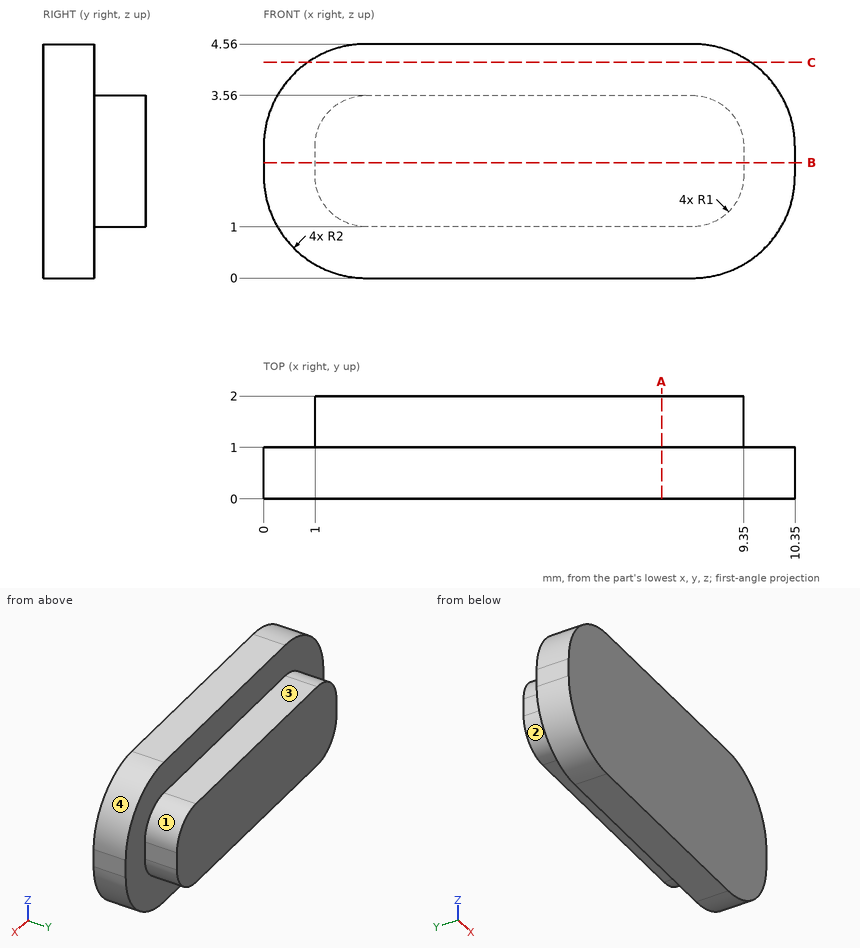
Print and shaded views of the part. All mm, measured from the part's lowest x, y and z. A direction names the side the tool comes from. Coordinates: 2 decimals unless noted, no trailing zeros. Order: outer loops, then holes, each group sorted by start corner. A loop starts at its lowest first (then second) coordinate and runs counter-clockwise, first axis right, second up. Notation, with made-up numbers: (44.5, -29) - (99.5, -29) arc R24 cw to (99.5, -1) - close; hole circle Ø8 at (83.5, -32.75). An arc over 180 degrees is marked (long way). Return JSON: item names as keys, results as strings. Group by question number.
Item 1: Cut at A-A (x = 7.75). List the corners of the cut face in (y, z), plus the area to 3 significant figures.
Item 2: Cut at C-C (z = 4.2). List the corners of the cut face in (x, y).
Item 3: Which spindle directions (+Z, -Z, +X, -X, +Y, -Y) get a long thin tool onto all of the face, cutting with end or side? Do the marked faces 1, 2, 3 and 4. Say none if no direction does.
Item 4: Drill centre lines: probe 1 along Y at (x, z) = (6.25, 3.7); probe 2 along X at (y, z) = (1.45, 2.35); probe 3 along Z at (x, y) = (3.25, 1.6). Where is each one in solid material? Low to high. Write a range as from..to.
Item 5: Cut at B-B (z = 2.25). List the corners of the cut face in (x, y), plus the area to 3 significant figures.
Item 6: Pin check, flat tip, straight feed: pin 1 (0.8 mm diameter, centred on x = 5.5, y = 1.5, fed in from +Z). Stop position of the tip, or through.
Check values:
{
 "1": {"outline": "(0, 0) - (1, 0) - (1, 1) - (2, 1) - (2, 3.56) - (1, 3.56) - (1, 4.56) - (0, 4.56) - close", "area": "7.12 mm2"},
 "2": {"outline": "(0.86, 0) - (9.49, 0) - (9.49, 1) - (0.86, 1) - close"},
 "3": {"face 1": "+Z, +X, +Y", "face 2": "-Z, -X, +Y", "face 3": "+Z, +X, -X, +Y", "face 4": "+Z, +X, +Y, -Y"},
 "4": {"probe 1": "y = 0..1", "probe 2": "x = 1..9.35", "probe 3": "z = 1..3.56"},
 "5": {"outline": "(0, 0) - (10.35, 0) - (10.35, 1) - (9.35, 1) - (9.35, 2) - (1, 2) - (1, 1) - (0, 1) - close", "area": "18.7 mm2"},
 "6": {"pin 1": "stops at z = 3.56"}
}
